For this review, take the finished solid that the model builds, in its own axes (mm). Face numbers are marked on the shaded views. A direction names the side the tool comes from. Coordinates: 2 decimals unless noted, no trailing zeros. Order: outer loops, then holes, each group sorted by start corner. A loop starts at its lowest first (then second) coordinate and runs counter-clockwise, first axis right, second up. Notation, with made-up numbers: (71, 62.5) -> (87, 62.5) arc R22 ccw to (87, 89.5) -> close; hole circle Ø1 at (11.5, 42). An arc over 180 degrees is marked (long way). Return JSON: item names as keys, results as strings. Group by question number.
Item 1: Take a section at D-D (z = 10). Write out the cut boundary in (x, y), then the cut area to 3 significant figures.
Item 2: Take a section at A-A (z = -13.75). Write out the cut boundary in (x, y).
Item 3: For line 1 along Z through (x, y) = (-12, 9); line 2 along Y through (x, z) = (14, 13.95); line 3 along Z through (x, y) = (12, 4), list the stretches that pass through material, from the lowest coordinate up.
Item 4: Take a section at B-B (y = 10.75). Write out the cut boundary in (x, z).
Item 5: Draft analysis for pull direction X (two halves, no side actions). For the marked faces 1, 2 and 3, state which applies: +X half, -X half, draft (parallel to the pull), parting line (faces both ways), or undercut.
Item 6: Machinability: for the marked faces 4, 5, 6, 7 and 8, which of the approach directions +Z, -Z, +X, -X, +Y, -Y give a long, thin tool a straight path to every point of the face, cutting with its end or side? Answer none if there is none.
Item 7: Take a section at C-C (x = 0). Write out the cut boundary in (y, z), then the cut area to 3 significant figures.
Item 8: Insertion check: pin 1 (4 mm diameter, centred on x = 0, z = -10, fed in from +Y); pin 2 (1 mm diameter, centred on x = 13, z = 3.5, fed in from -Y); pin 3 (2.5 mm diameter, centred on y = 9, z = -13.75, fed in from +X); pin 4 (2 mm diameter, centred on y = 9, z = 13.95, fed in from -X). Each pin has a flat end and moves straight along its axis. Give the tip position at first contact, or say it passes through.
```python
from build123d import *

# Parameters (mm, degrees)
SKETCH_1_W          = 56
SKETCH_1_H          = 36
EXTRUDE_1_DEPTH     = 2.5
SKETCH_2_W          = 12
SKETCH_2_H          = 6
EXTRUDE_2_DEPTH     = 12
SKETCH_3_R          = 0.95
CUT_EXTRUDE_1_DEPTH = 54.275228765
SKETCH_4_R          = 1.75
CUT_EXTRUDE_2_DEPTH = 36.383612026


with BuildPart() as part:
    # 草图1 → 凸台-拉伸1 (new body)
    with BuildSketch(Plane(origin=(0, 0, 0), x_dir=(1, 0, 0), z_dir=(0, 1, 0))):
        Rectangle(SKETCH_1_W, SKETCH_1_H)
    extrude(amount=EXTRUDE_1_DEPTH)

    # 草图2 → 凸台-拉伸2 (add)
    with BuildSketch(Plane(origin=(0, 2.5, 0), x_dir=(1, 0, 0), z_dir=(0, 1, 0))):
        with Locations((14, 14.8)):
            Rectangle(SKETCH_2_W, SKETCH_2_H)
        with Locations((14, -15)):
            Rectangle(SKETCH_2_W, SKETCH_2_H)
    extrude_2 = extrude(amount=EXTRUDE_2_DEPTH)

    # 草图3 → 切除-拉伸1 (cut, through all)
    with BuildSketch(Plane(origin=(20, 0, 0), x_dir=(0, 0, -1), z_dir=(1, 0, 0))):
        with Locations((-13.95, 9)):
            Circle(SKETCH_3_R)
        with Locations((13.75, 9)):
            Circle(SKETCH_3_R)
    cut_extrude_1 = extrude(amount=-CUT_EXTRUDE_1_DEPTH, mode=Mode.SUBTRACT)

    # 镜向1: 凸台-拉伸2, 切除-拉伸1 across plane
    add(extrude_2.mirror(Plane(origin=(0, 0, 0), x_dir=(0, 0, 1), z_dir=(1, 0, 0))))
    add(cut_extrude_1.mirror(Plane(origin=(0, 0, 0), x_dir=(0, 0, 1), z_dir=(1, 0, 0))), mode=Mode.SUBTRACT)

    # 草图4 → 切除-拉伸2 (cut, through all)
    with BuildSketch(Plane(origin=(0, 2.5, 0), x_dir=(1, 0, 0), z_dir=(0, 1, 0))):
        with Locations(Location((0, -10, 0), (0, 0, 270))):
            Circle(SKETCH_4_R)
        with Locations(Location((0, 10, 0), (0, 0, 270))):
            Circle(SKETCH_4_R)
    extrude(amount=-CUT_EXTRUDE_2_DEPTH, mode=Mode.SUBTRACT)


solid = part.part
```
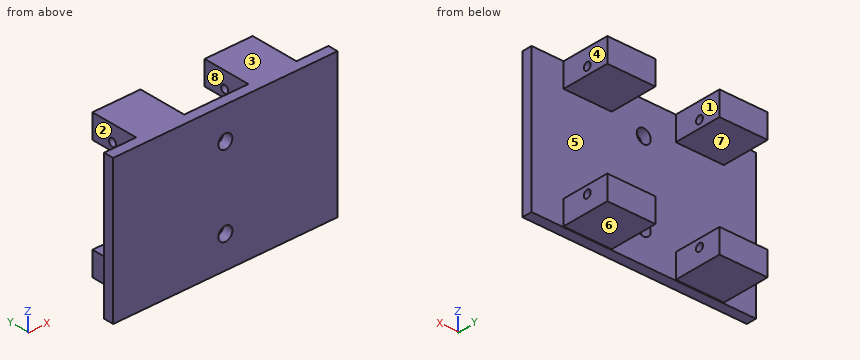
Findings below:
{
 "1": {"outline": "(-28, 0) -> (-1.75, 0) -> (-1.75, 2.5) -> (-28, 2.5) -> close; (1.75, 0) -> (28, 0) -> (28, 2.5) -> (1.75, 2.5) -> close", "area": "131 mm2"},
 "2": {"outline": "(-28, 0) -> (28, 0) -> (28, 2.5) -> (20, 2.5) -> (20, 8.05) -> (8, 8.05) -> (8, 2.5) -> (-8, 2.5) -> (-8, 8.05) -> (-20, 8.05) -> (-20, 2.5) -> (-28, 2.5) -> close; (-20, 9.95) -> (-8, 9.95) -> (-8, 14.5) -> (-20, 14.5) -> close; (8, 9.95) -> (20, 9.95) -> (20, 14.5) -> (8, 14.5) -> close"},
 "3": {"line 1": "z = -17.8 to -14.7, -12.8 to -11.8, 12 to 13, 14.9 to 18", "line 2": "y = 0 to 8.05, 9.95 to 14.5", "line 3": "z = -17.8 to -11.8, 12 to 18"},
 "4": {"outline": "(-20, -17.8) -> (-8, -17.8) -> (-8, -11.8) -> (-20, -11.8) -> close; (-20, 12) -> (-8, 12) -> (-8, 18) -> (-20, 18) -> close; (8, -17.8) -> (20, -17.8) -> (20, -11.8) -> (8, -11.8) -> close; (8, 12) -> (20, 12) -> (20, 18) -> (8, 18) -> close"},
 "5": {"face 1": "undercut", "face 2": "-X half", "face 3": "draft"},
 "6": {"face 4": "+Z, -Z, +X, +Y", "face 5": "+Y", "face 6": "-Z, +X, -X, +Y", "face 7": "+X, -X, +Y", "face 8": "+Z, -Z, +Y"},
 "7": {"outline": "(0, -18) -> (2.5, -18) -> (2.5, -11.75) -> (0, -11.75) -> close; (0, -8.25) -> (2.5, -8.25) -> (2.5, 8.25) -> (0, 8.25) -> close; (0, 11.75) -> (2.5, 11.75) -> (2.5, 18) -> (0, 18) -> close", "area": "72.5 mm2"},
 "8": {"pin 1": "stops at y = 2.5", "pin 2": "stops at y = 0", "pin 3": "stops at x = 20", "pin 4": "stops at x = -20"}
}
